The drawing under review shows one solid part. Ordinate dimensions are in mm from its lowest x, y, z. A direction names the side the tool comes from. Coordinates: 2 decimals unless noted, no trailing zeros. Write each loop counter-clockwise with the first axis right and the second up, starting at its lowest first coordinate (ties: lowest second). Pieces come first, ordered by that corner, then holes.
Q1. To check wall thickness, follow probe 1 along X at (y, z) = (147, 173); probe 2 along Z at (x, y) = (377, 161.5). State the ranges of each line that lie inside material, in increasing order.
Q2. The part is to be moulded in two halves that separate along Z. For the marked faces 3, 4 and 5, say which applies: +Z half, -Z half, draft (parallel to the pull), parting line (faces both ways), or undercut.
Q3. Add section B-B, the plane x = 390.5. Give the boundary of the cut face in (y, z), plus the area to 3 significant figures.
Q4. Machinability: for the marked faces 1 and 2, which of the approach directions +Z, -Z, +X, -X, +Y, -Y give a long, thin tool a straight path to every point of the face, cutting with its end or side? Answer none if there is none.
Q5. Add section C-C, the plane y = 78.5. Give the boundary of the cut face in (x, z).
Q6. Add section A-A, the plane z = 154. Give the boundary of the cut face in (x, y), plus the area to 3 significant figures.
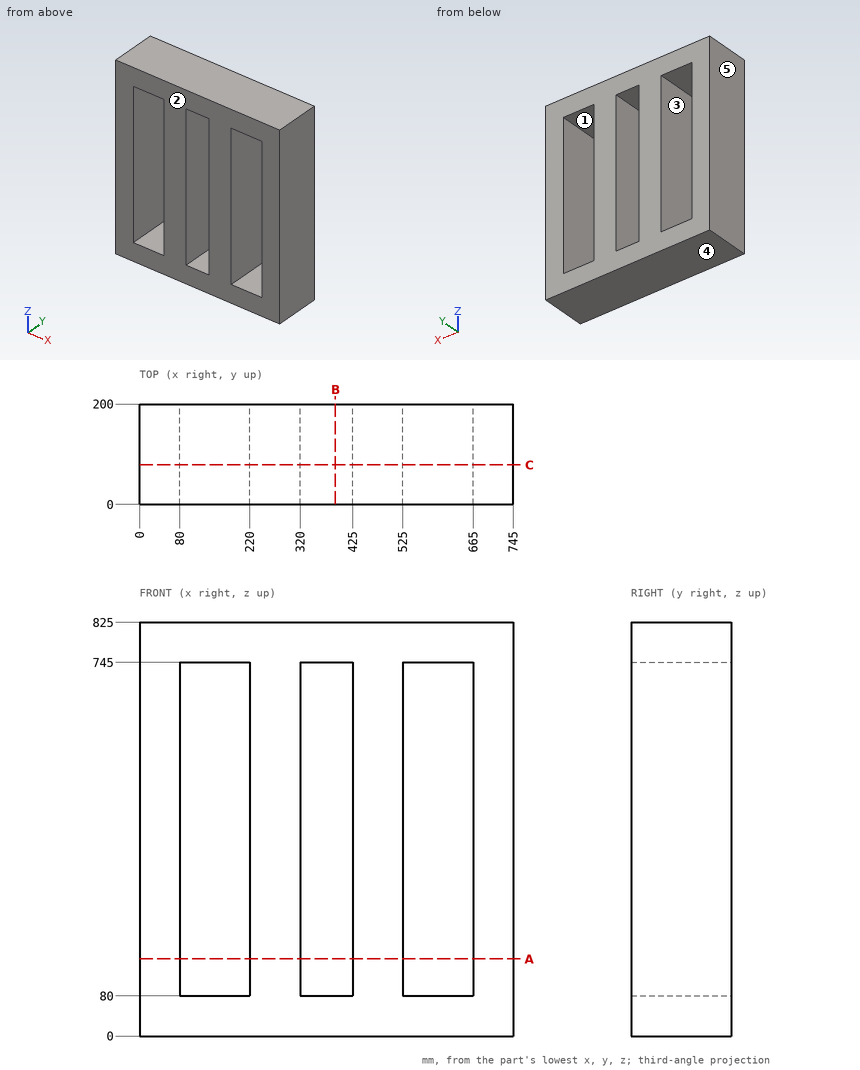
Here are the results:
1. probe 1: x = 0 to 80, 220 to 320, 425 to 525, 665 to 745
1. probe 2: z = 0 to 80, 745 to 825
2. face 3: undercut
2. face 4: -Z half
2. face 5: draft
3. outline: (0, 0) - (200, 0) - (200, 80) - (0, 80) - close; (0, 745) - (200, 745) - (200, 825) - (0, 825) - close
3. area: 32,000 mm2
4. face 1: +Y, -Y
4. face 2: +Z, -Z, +X, -X, -Y
5. outline: (0, 0) - (745, 0) - (745, 825) - (0, 825) - close; hole (80, 80) - (220, 80) - (220, 745) - (80, 745) - close; hole (320, 80) - (425, 80) - (425, 745) - (320, 745) - close; hole (525, 80) - (665, 80) - (665, 745) - (525, 745) - close
6. outline: (0, 0) - (80, 0) - (80, 200) - (0, 200) - close; (220, 0) - (320, 0) - (320, 200) - (220, 200) - close; (425, 0) - (525, 0) - (525, 200) - (425, 200) - close; (665, 0) - (745, 0) - (745, 200) - (665, 200) - close
6. area: 72,000 mm2
